from build123d import *

# Parameters (mm, degrees)
SKETCH1_W           = 170.000000106
SKETCH1_H           = 170.000000106
BOSS_EXTRUDE1_DEPTH = 2
SKETCH2_W           = 128.519017825
SKETCH2_H           = 5.853406533
BOSS_EXTRUDE2_DEPTH = 40
SKETCH3_W           = 84.023612157
SKETCH3_H           = 84.023612156
BOSS_EXTRUDE3_DEPTH = 40
SKETCH4_W           = 25.047517012
SKETCH4_H           = 14.903147005
SKETCH4_W_2         = 19.766346878
SKETCH4_H_2         = 22.517192253
SKETCH4_W_3         = 18.992337586
BOSS_EXTRUDE4_DEPTH = 30
SKETCH5_W           = 21.301196701
SKETCH5_H           = 18.135167802
BOSS_EXTRUDE5_DEPTH = 20
SKETCH6_W           = 33.473309102
SKETCH6_H           = 11.440505981
BOSS_EXTRUDE6_DEPTH = 25
SKETCH7_W           = 16.858518609
SKETCH7_H           = 17.730572085
SKETCH7_W_2         = 51.529446996
SKETCH7_H_2         = 10.618502019
BOSS_EXTRUDE7_DEPTH = 30.95
SKETCH8_W           = 37.52039774
SKETCH8_H           = 34.539531191
SKETCH8_W_2         = 7.616701468
SKETCH8_H_2         = 90.426961443
BOSS_EXTRUDE8_DEPTH = 10
SKETCH9_R           = 2.032
CUT_EXTRUDE1_DEPTH  = 10


with BuildPart() as part:
    # Sketch1 → Boss-Extrude1 (new body)
    with BuildSketch(Plane(origin=(0, 0, 0), x_dir=(1, 0, 0), z_dir=(0, 1, 0))):
        Rectangle(SKETCH1_W, SKETCH1_H)
    extrude(amount=BOSS_EXTRUDE1_DEPTH)

    # Sketch2 → Boss-Extrude2 (add)
    with BuildSketch(Plane(origin=(0, 2, 0), x_dir=(1, 0, 0), z_dir=(0, 1, 0))):
        with Locations((10.509835463, -56.422676592)):
            Rectangle(SKETCH2_W, SKETCH2_H)
        with Locations((10.509835463, -64.84262126)):
            Rectangle(SKETCH2_W, SKETCH2_H)
    extrude(amount=BOSS_EXTRUDE2_DEPTH)

    # Sketch3 → Boss-Extrude3 (add)
    with BuildSketch(Plane(origin=(0, 2, 0), x_dir=(1, 0, 0), z_dir=(0, 1, 0))):
        with Locations((17.355096342, -2.434194161)):
            Rectangle(SKETCH3_W, SKETCH3_H)
    extrude(amount=BOSS_EXTRUDE3_DEPTH)

    # Sketch4 → Boss-Extrude4 (add)
    with BuildSketch(Plane(origin=(0, 2, 0), x_dir=(1, 0, 0), z_dir=(0, 1, 0))):
        with Locations((-59.772791477, 77.548426551)):
            Rectangle(SKETCH4_W, SKETCH4_H)
        with Locations((-34.352625517, 73.741403926)):
            Rectangle(SKETCH4_W_2, SKETCH4_H_2)
        with Locations((-12.41080084, 73.741403926)):
            Rectangle(SKETCH4_W_3, SKETCH4_H_2)
    extrude(amount=BOSS_EXTRUDE4_DEPTH)

    # Sketch5 → Boss-Extrude5 (add)
    with BuildSketch(Plane(origin=(0, 2, 0), x_dir=(1, 0, 0), z_dir=(0, 1, 0))):
        with Locations((11.275402632, 75.932416152)):
            Rectangle(SKETCH5_W, SKETCH5_H)
    extrude(amount=BOSS_EXTRUDE5_DEPTH)

    # Sketch6 → Boss-Extrude6 (add)
    with BuildSketch(Plane(origin=(0, 2, 0), x_dir=(1, 0, 0), z_dir=(0, 1, 0))):
        with Locations((42.922894873, 79.279747063)):
            Rectangle(SKETCH6_W, SKETCH6_H)
    extrude(amount=BOSS_EXTRUDE6_DEPTH)

    # Sketch7 → Boss-Extrude7 (add)
    with BuildSketch(Plane(origin=(0, 2, 0), x_dir=(1, 0, 0), z_dir=(0, 1, 0))):
        with Locations((76.570740749, 76.134714011)):
            Rectangle(SKETCH7_W, SKETCH7_H)
        with Locations((43.928389082, -79.690749044)):
            Rectangle(SKETCH7_W_2, SKETCH7_H_2)
    extrude(amount=BOSS_EXTRUDE7_DEPTH)

    # Sketch8 → Boss-Extrude8 (add)
    with BuildSketch(Plane(origin=(0, 2, 0), x_dir=(1, 0, 0), z_dir=(0, 1, 0))):
        with Locations((-49.174587618, -20.138415223)):
            Rectangle(SKETCH8_W, SKETCH8_H)
        with Locations((-77.515242813, -1.936857576)):
            Rectangle(SKETCH8_W_2, SKETCH8_H_2)
    extrude(amount=BOSS_EXTRUDE8_DEPTH)

    # Sketch9 → Cut-Extrude1 (cut)
    with BuildSketch(Plane(origin=(0, 2, 0), x_dir=(1, 0, 0), z_dir=(0, 1, 0))):
        with Locations(Location((-78.650000053, 74.840000053, 0), (0, 0, 270))):
            Circle(SKETCH9_R)
        with Locations(Location((78.829999947, 51.980000053, 0), (0, 0, 270))):
            Circle(SKETCH9_R)
        with Locations(Location((78.829999947, -80.099999947, 0), (0, 0, 270))):
            Circle(SKETCH9_R)
        with Locations(Location((-78.650000053, -80.099999947, 0), (0, 0, 270))):
            Circle(SKETCH9_R)
    extrude(amount=-CUT_EXTRUDE1_DEPTH, mode=Mode.SUBTRACT)


solid = part.part
Read the model definition and answer for the solid it produces. Units are mm, in the model's axes. A direction names the side the tool comes from. Give positions to 0.01 mm unless a question says otherwise; leave off trailing zeros. Write each loop counter-clockwise with the first axis right and the second up, starting at its lowest first coordinate (ties: lowest second). Pieces come first, ordered by that corner, then holes. Notation, with made-up numbers: (-34, -29.5) - (-20, -29.5) arc R10 cw to (-20, -25.5) - close; hole circle Ø7 at (-32, 20.5). An arc over 180 degrees is marked (long way). Answer in a Markdown table with one row per item. Add a question column.
Item 1: Section D-D, the plane z = 28 is taken. Write down the section's boundary in (x, y), and give its area (3 significant figures).
Item 2: A tool of negligible diameter and unlimited length cuts with its end or side. For faces 4 (the face through (-34, 17, -62.483)), 5 (the face through (59.66, 14, -79)), 6 (the face through (-53.75, 22, 56)), from which of +Z, -Z, +X, -X, +Y, -Y can it reach the whole face along a straight path? Write none if from no direction.
Item 3: Flat-ended cylindrical pins translate along their axes: P1, Ø4, axis at y = 8, z = 28, coming from the +X side; P2, Ø20, axis at x = -10, y = 29.5, coming from the +Z side; P3, Ø5.5, axis at x = 49, z = -80.5, coming from the +Y side. Find the tip coordinate at first contact, or state that the pin passes through.
Item 4: Determine the mould class of faces 1 (the face through (-30.414, 7, 20)), 2 (the face through (37, 14, 85)), 3 (the face through (74.769, 22, 65)) for opening direction Z: pulls with the +Z half, pulls with the -Z half, needs draft (parallel to the pull), parting line crosses it, or undercut.
Item 5: Section C-C, the plane z = -51.98 is taken. Write down the section's boundary in (x, y).
Item 6: Find the intervals of material crossed by L1, parallel to Z at x = -78.65, y = 1.1; L2, parallel to Z at x = 40.5, y = 38.5; L3, parallel to Z at x = 38.5, y = 20, in increasing order.
Item 7: Section A-A, the plane y = 29 is taken. Count the separate pieces of the cut face and the enclosed holes in it, and give its area (3 significant figures).
Item 8: Section B-B, the plane x = 78.83 is taken. Write down the section's boundary in (y, z).
Recorded:
| question | item | result |
|---|---|---|
| 1 | outline | (-85, 0) - (85, 0) - (85, 2) - (59.37, 2) - (59.37, 42) - (-24.66, 42) - (-24.66, 2) - (-30.41, 2) - (-30.41, 12) - (-67.93, 12) - (-67.93, 2) - (-73.71, 2) - (-73.71, 12) - (-81.32, 12) - (-81.32, 2) - (-85, 2) - close |
| 1 | area | 4,150 mm2 |
| 2 | face 4 | +X, -X, +Y |
| 2 | face 5 | -Z, +Y |
| 2 | face 6 | +Z, -X, +Y |
| 3 | P1 | stops at x = 59.37 |
| 3 | P2 | stops at z = 67.77 |
| 3 | P3 | stops at y = 27 |
| 4 | face 1 | undercut |
| 4 | face 2 | pulls with the +Z half |
| 4 | face 3 | needs draft |
| 5 | outline | (-85, 0) - (76.8, 0) - (76.8, 2) - (-85, 2) - close; (80.86, 0) - (85, 0) - (85, 2) - (80.86, 2) - close |
| 6 | L1 | z = -85 to -76.87, -72.81 to 78.07, 82.13 to 85 |
| 6 | L2 | z = -39.58 to 44.45, 53.5 to 59.35, 61.92 to 67.77 |
| 6 | L3 | z = -85 to -73.56, -39.58 to 44.45, 53.5 to 59.35, 61.92 to 67.77, 74.38 to 85 |
| 7 | separate pieces | 8 |
| 7 | enclosed holes | 0 |
| 7 | area | 10,700 mm2 |
| 8 | outline | (0, -85) - (32.95, -85) - (32.95, -67.27) - (2, -67.27) - (2, -54.01) - (0, -54.01) - close; (0, -49.95) - (2, -49.95) - (2, 78.07) - (0, 78.07) - close; (0, 82.13) - (2, 82.13) - (2, 85) - (0, 85) - close |
